Geometry check sheet. Reference: the model listing, model coordinates, mm. Round coordinates to 2 decimals unless told otherwise and drop trailing zeros. Loops run counter-clockwise (first coordinate to the right, second up) from the corner with the lowest first, then second, coordinate; pieces in that order, holes last. Notation, with made-up numbers: M 13,7 L 49,7 A27 ccw 49,29 Z; hole C -11.5,4 d6. An arc over 180 degrees is marked long. Write item = value, one per line.
from build123d import *

# Parameters (mm, degrees)
SCHIZZO2_W                   = 118
SCHIZZO2_H                   = 96
ESTRUSIONE_ESTRUSIONE1_DEPTH = 20
ESTRUSIONE_ESTRUSIONE2_DEPTH = 170


with BuildPart() as part:
    # Schizzo2 → Estrusione-Estrusione1 (new body)
    with BuildSketch(Plane(origin=(0, 0, 0), x_dir=(1, 0, 0), z_dir=(0, 1, 0))):
        Rectangle(SCHIZZO2_W, SCHIZZO2_H)
    extrude(amount=ESTRUSIONE_ESTRUSIONE1_DEPTH)

    # Schizzo3 → Estrusione-Estrusione2 (add)
    with BuildSketch(Plane(origin=(0, 0, 0), x_dir=(1, 0, 0), z_dir=(0, 1, 0))):
        with BuildLine():
            Line((-49.216117819, 28), (-54, 28))
            Line((-54, 28), (-54, 43))
            Line((-54, 43), (-49.216117819, 43))
            ThreePointArc((-49.216117819, 43), (-44, 35.5), (-49.216117819, 28))
        make_face()
    extrude(amount=ESTRUSIONE_ESTRUSIONE2_DEPTH)

    # Specchia3: part across plane


with BuildPart() as part_1:
    add(part.part)
    add(part.part.mirror(Plane(origin=(-59, 20, 48), x_dir=(1, 0, 0), z_dir=(0, 0, -1))))

    # Specchia2: part across plane


with BuildPart() as part_2:
    add(part_1.part)
    add(part_1.part.mirror(Plane(origin=(59, 20, -48), x_dir=(0, 0, 1), z_dir=(-1, 0, 0))))


solid = part_2.part
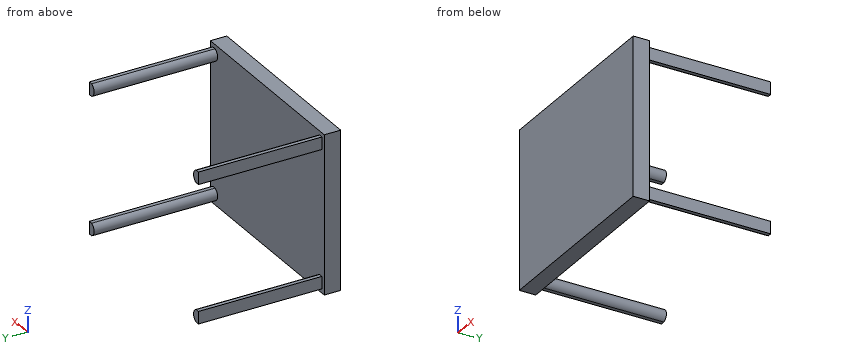
(1) Material ranges on line 1 along Y through (x, z) = (111, 115), recorded low to high. Write a range as from..to.
Result set:
line_1 = 0..20
(2) Sectioned sample at B-B on z = -35.5. Record the cut outline in (x, y), then the cut area to 3 significant figures.
Result set:
outline = M -59,0 L 177,0 L 177,20 L 172,20 L 172,170 L 162,170 L 162,20 L -44,20 L -44,170 L -54,170 L -54,20 L -59,20 Z
area = 7,720 mm2
(3) Sectioned sample at D-D on z = 64.5. Record the cut outline in (x, y).
Result set:
outline = M -59,0 L 177,0 L 177,20 L -59,20 Z
(4) Sectioned sample at A-A on y = 154. Record the cut outline in (x, z), then the cut area to 3 significant figures.
Result set:
outline = M -54,-43 L -49.22,-43 A8 ccw -49.22,-28 L -54,-28 Z; M -54,124 L -49.22,124 A8 ccw -49.22,139 L -54,139 Z; M 167.22,-43 L 172,-43 L 172,-28 L 167.22,-28 A8 ccw Z; M 167.22,124 L 172,124 L 172,139 L 167.22,139 A8 ccw Z
area = 515 mm2
(5) Depth check by flat-ended pin: pin 1 Ø2.5 at (x, y) = (-52.5, 63) entering from +Z; pin 2 Ø1.4 at (x, y) = (-51.5, 76.5) entering from -Z; pin 3 Ø7.5 at (y, z) = (108, -36.5) entering from -X. Enter the tip coordinate at first touch or a pass-through.
Result set:
pin_1 = 139
pin_2 = -43
pin_3 = -54
(6) Sectioned sample at C-C on x = -22. Record the cut outline in (y, z).
Result set:
outline = M 0,-48 L 20,-48 L 20,144 L 0,144 Z
